Build history of the part. All positions in model axes, mm. A direction names the side the tool comes from. Give positions to 0.01 mm unless a question says otherwise; leave off trailing zeros. Loops run counter-clockwise (first coordinate to the right, second up) from the corner with the lowest first, then second, coordinate; pieces in that order, holes last. Notation, with made-up numbers: (11.25, 77.5) -> (63.25, 77.5) arc R27 cw to (63.25, 107.5) -> close; hole circle Ø1 at (63, 5.25). An arc over 180 degrees is marked (long way). Answer in a Markdown table with one row per item. Add a question column.
from build123d import *

# Parameters (mm, degrees)
BOSS_EXTRUDE1_DEPTH = 3


with BuildPart() as part:
    # Sketch1 → Boss-Extrude1 (new body)
    with BuildSketch(Plane.XY):
        with BuildLine():
            Line((-55.5, -50), (-40, -50))
            Line((-40, -50), (-40, -53))
            Line((-40, -53), (-20, -53))
            Line((-20, -53), (-20, -50))
            Line((-20, -50), (-10, -50))
            Line((-10, -50), (-10, -53))
            Line((-10, -53), (10, -53))
            Line((10, -53), (10, -50))
            Line((10, -50), (20, -50))
            Line((20, -50), (20, -53))
            Line((20, -53), (40, -53))
            Line((40, -53), (40, -50))
            Line((40, -50), (40.851130485, -50))
            ThreePointArc((40.851130485, -50), (45.851130485, -45), (50.851130485, -50))
            Line((50.851130485, -50), (55.5, -50))
            Line((55.5, -50), (55.5, -35))
            Line((55.5, -35), (58.5, -35))
            Line((58.5, -35), (58.5, -15))
            Line((58.5, -15), (55.5, -15))
            Line((55.5, -15), (55.5, -10))
            Line((55.5, -10), (58.5, -10))
            Line((58.5, -10), (58.5, 10))
            Line((58.5, 10), (55.5, 10))
            Line((55.5, 10), (55.5, 15))
            Line((55.5, 15), (58.5, 15))
            Line((58.5, 15), (58.5, 35))
            Line((58.5, 35), (55.5, 35))
            Line((55.5, 35), (55.5, 50))
            Line((55.5, 50), (-55.5, 50))
            Line((-55.5, 50), (-55.5, 35))
            Line((-55.5, 35), (-58.5, 35))
            Line((-58.5, 35), (-58.5, 15))
            Line((-58.5, 15), (-55.5, 15))
            Line((-55.5, 15), (-55.5, 10))
            Line((-55.5, 10), (-58.5, 10))
            Line((-58.5, 10), (-58.5, -10))
            Line((-58.5, -10), (-55.5, -10))
            Line((-55.5, -10), (-55.5, -15))
            Line((-55.5, -15), (-58.5, -15))
            Line((-58.5, -15), (-58.5, -35))
            Line((-58.5, -35), (-55.5, -35))
            Line((-55.5, -35), (-55.5, -50))
        make_face()
        with BuildLine():
            Line((-40, 35), (-10, 35))
            ThreePointArc((-10, 35), (-5, 30), (-10, 25))
            Line((-10, 25), (-40, 25))
            ThreePointArc((-40, 25), (-45, 30), (-40, 35))
        make_face(mode=Mode.SUBTRACT)
        with BuildLine():
            Line((10, 35), (40, 35))
            ThreePointArc((40, 35), (45, 30), (40, 25))
            Line((40, 25), (10, 25))
            ThreePointArc((10, 25), (5, 30), (10, 35))
        make_face(mode=Mode.SUBTRACT)
        with BuildLine():
            Line((-7.5, -15), (-7.5, 15))
            ThreePointArc((-7.5, 15), (0, 22.5), (7.5, 15))
            Line((7.5, 15), (7.5, -15))
            ThreePointArc((7.5, -15), (0, -22.5), (-7.5, -15))
        make_face(mode=Mode.SUBTRACT)
        with BuildLine():
            Line((-40, -5), (-15, -5))
            ThreePointArc((-15, -5), (-10, -10), (-15, -15))
            Line((-15, -15), (-40, -15))
            ThreePointArc((-40, -15), (-45, -10), (-40, -5))
        make_face(mode=Mode.SUBTRACT)
        with BuildLine():
            Line((15, -5), (40, -5))
            ThreePointArc((40, -5), (45, -10), (40, -15))
            Line((40, -15), (15, -15))
            ThreePointArc((15, -15), (10, -10), (15, -5))
        make_face(mode=Mode.SUBTRACT)
        with BuildLine():
            Line((-40, -36.056835362), (-20, -36.056835362))
            ThreePointArc((-20, -36.056835362), (-17.5, -38.556835362), (-20, -41.056835362))
            Line((-20, -41.056835362), (-40, -41.056835362))
            ThreePointArc((-40, -41.056835362), (-42.5, -38.556835362), (-40, -36.056835362))
        make_face(mode=Mode.SUBTRACT)
        with BuildLine():
            Line((39.496814851, -41.056835362), (19.496814851, -41.056835362))
            ThreePointArc((19.496814851, -41.056835362), (16.996814851, -38.556835362), (19.496814851, -36.056835362))
            Line((19.496814851, -36.056835362), (39.496814851, -36.056835362))
            ThreePointArc((39.496814851, -36.056835362), (41.996814851, -38.556835362), (39.496814851, -41.056835362))
        make_face(mode=Mode.SUBTRACT)
    extrude(amount=BOSS_EXTRUDE1_DEPTH)


solid = part.part
(1) Two-plate mould, pull along X, no slides. Class faces 4 (the flat face through (-58.5, 25, 1)), 5 (the flat face through (53, -50, 1)), 6 (the flat face through (30, -41.057, 1)): released by +X, released by -X, zero draft, split by the parting line, or undercut.
(2) Saw through at C-C, the plane x = 0. List the corners of the cut face in (y, z), then the cut area to 3 significant figures.
(3) Saw through at B-B, the plane x = 36. List the corners of the cut face in (y, z), then the cut area to 3 significant figures.
(4) Saw through at A-A, the plane y = 19.5. List the corners of the cut face in (x, z), then the cut area to 3 significant figures.
(5) Saw through at D-D, the plane z = 2.55. State how many separate pieces and enclosed holes the cut face has, then the cut area to 3 significant figures.
(6) Wall check: line 1 along Y through (x, z) = (26, 0.9); line 2 along X through (y, z) = (-10.5, 0.4); line 3 along X through (y, z) = (30, 1.45). Give the ranges that are in metal, low to high. Write a range as from..to.
(7) 3-axis set-ups, long thin cutter, end or side, ignore diameter. For faces 1 (the cylindrical face through (0.16, -22.5, 1.48)), 2 (the flat face through (57, -35, 1)), 3 (the flat face through (-57, -10, 1)): which of +Z, -Z, +X, -X, +Y, -Y reach the whole face in a straight line?
(8) Flat gauge pins, fed straight in: pin 1 Ø1.5 at (y, z) = (-12, 2) entering from -X; pin 2 Ø0.9 at (x, z) = (-57.5, 1.5) entering from +Y; pin 3 Ø1.5 at (x, z) = (-45, 2) entering from -Y. Where does each tip first touch, or does it go through?
Worked answers:
| question | item | result |
|---|---|---|
| 1 | face 4 | released by -X |
| 1 | face 5 | zero draft |
| 1 | face 6 | undercut |
| 2 | outline | (-53, 0) -> (-22.5, 0) -> (-22.5, 3) -> (-53, 3) -> close; (22.5, 0) -> (50, 0) -> (50, 3) -> (22.5, 3) -> close |
| 2 | area | 174 mm^2 |
| 3 | outline | (-53, 0) -> (-41.06, 0) -> (-41.06, 3) -> (-53, 3) -> close; (-36.06, 0) -> (-15, 0) -> (-15, 3) -> (-36.06, 3) -> close; (-5, 0) -> (25, 0) -> (25, 3) -> (-5, 3) -> close; (35, 0) -> (50, 0) -> (50, 3) -> (35, 3) -> close |
| 3 | area | 234 mm^2 |
| 4 | outline | (-58.5, 0) -> (-6, 0) -> (-6, 3) -> (-58.5, 3) -> close; (6, 0) -> (58.5, 0) -> (58.5, 3) -> (6, 3) -> close |
| 4 | area | 315 mm^2 |
| 5 | separate pieces | 1 |
| 5 | enclosed holes | 7 |
| 5 | area | 9,320 mm^2 |
| 6 | line 1 | -53..-41.06, -36.06..-15, -5..25, 35..50 |
| 6 | line 2 | -55.5..-44.97, -10.03..-7.5, 7.5..10.03, 44.97..55.5 |
| 6 | line 3 | -58.5..-45, -5..5, 45..58.5 |
| 7 | face 1 | +Z, -Z |
| 7 | face 2 | +Z, -Z, +X, -Y |
| 7 | face 3 | +Z, -Z, -X |
| 8 | pin 1 | x = -55.5 |
| 8 | pin 2 | y = 35 |
| 8 | pin 3 | y = -50 |
